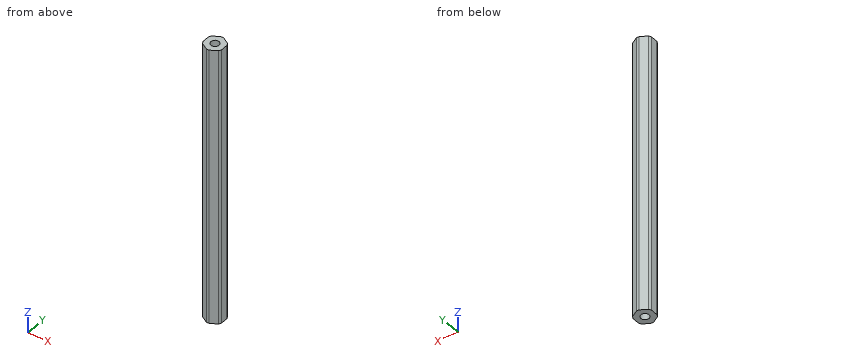
from build123d import *

# Parameters (mm, degrees)
SHAFT_BOSS_DEPTH                = 457.2
SKETCH2_R                       = 7.66445
SKETCH2_R_2                     = 5.12445
CUT_FOR_THUNDER_HEX_ROUND_DEPTH = 914.4
SKETCH3_R                       = 2.0955
CENTER_HOLE_CUT_DEPTH           = 914.4


with BuildPart() as part:
    # Sketch1 → Shaft Boss (new, symmetric)
    with BuildSketch(Plane.XY):
        Polygon((0, 5.499261314), (-4.7625, 2.749630657), (-4.7625, -2.749630657), (0, -5.499261314), (4.7625, -2.749630657), (4.7625, 2.749630657), align=None)
    extrude(amount=SHAFT_BOSS_DEPTH, both=True)

    # Sketch2 → Cut For Thunder Hex Round (cut)
    with BuildSketch(Plane(origin=(0, 0, -457.2), x_dir=(-1, 0, 0), z_dir=(0, 0, -1))):
        Circle(SKETCH2_R)
        Circle(SKETCH2_R_2, mode=Mode.SUBTRACT)
    extrude(amount=-CUT_FOR_THUNDER_HEX_ROUND_DEPTH, mode=Mode.SUBTRACT)

    # Sketch3 → Center Hole Cut (cut)
    with BuildSketch(Plane(origin=(0, 0, -457.2), x_dir=(-1, 0, 0), z_dir=(0, 0, -1))):
        Circle(SKETCH3_R)
    extrude(amount=-CENTER_HOLE_CUT_DEPTH, mode=Mode.SUBTRACT)

    # SurfaceCut1
    split(bisect_by=Plane(origin=(0, 0, 71.9105), x_dir=(-1, 0, 0), z_dir=(0, 0, -1)), keep=Keep.TOP)

    # SurfaceCut2
    split(bisect_by=Plane.XY.offset(-71.9105), keep=Keep.TOP)


solid = part.part
The listing builds one solid part. Answer for the finished solid, in the listing's coordinates (mm). Round coordinates to 2 decimals unless told otherwise and drop trailing zeros. Write each loop counter-clockwise with the first axis right and the second up, starting at its lowest first coordinate (ties: lowest second). Pieces come first, ordered by that corner, then holes. Notation, with made-up numbers: M -33.75,57.25 L -21.75,57.25 A9 ccw -21.75,73.25 Z; hole C 47.5,20 d3. An arc over 180 degrees is marked long. Write each question's results on one line, items separated by ' | '. Start each with the question number.
(1) The part is cut by section B-B, the plane z = 55.5. Write down the section's boundary in (x, y).
(2) Find the intervals of material crossed by line 1 (Y direction, x = -0.25, z = -26); line 2 (Y direction, x = -1.5, z = -42.5); line 3 (X direction, y = -0.5, z = 2.5), in increasing order.
(3) The part is cut by section A-A, the plane y = 0. Write down the section's boundary in (x, z).
(4) Each of these flat-tipped pins is pushed along its axis until it touches: P1, Ø2, axis at x = 1.5, z = 14, coming from the -Y side; P2, Ø4, axis at x = 0, y = 0, coming from the -Z side; P3, Ø3, axis at x = -3, z = -52, coming from the +Y side. Where does it stop, or does it pass through?
Worked answers:
1) outline: M -4.76,-1.89 A5.12 ccw -4.02,-3.18 L -0.74,-5.07 A5.12 ccw 0.74,-5.07 L 4.02,-3.18 A5.12 ccw 4.76,-1.89 L 4.76,1.89 A5.12 ccw 4.02,3.18 L 0.74,5.07 A5.12 ccw -0.74,5.07 L -4.02,3.18 A5.12 ccw -4.76,1.89 Z; hole C 0,0 d4.19
2) line 1: y = -5.12 to -2.08, 2.08 to 5.12 | line 2: y = -4.63 to -1.46, 1.46 to 4.63 | line 3: x = -4.76 to -2.03, 2.03 to 4.76
3) outline: M -4.76,-71.91 L -2.1,-71.91 L -2.1,71.91 L -4.76,71.91 Z; M 2.1,-71.91 L 4.76,-71.91 L 4.76,71.91 L 2.1,71.91 Z
4) P1: stops at y = -5.1 | P2: passes through | P3: stops at y = 4.63
